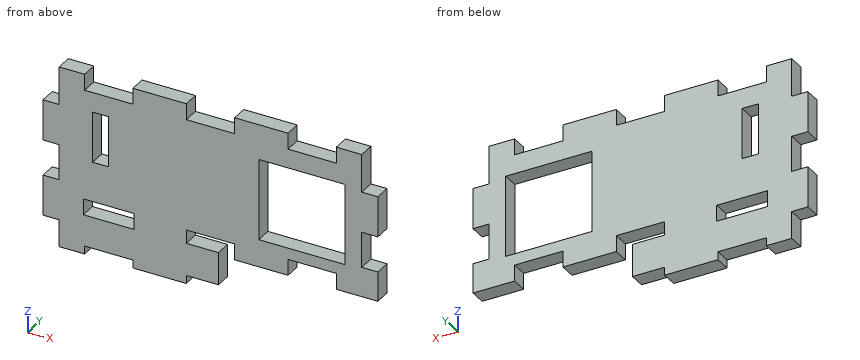
from build123d import *

# Parameters (mm, degrees)
BOTTOM_START                  = -0.928285838
BOTTOM_SIDE_PIECE_OUTLINE_W   = 3.175
BOTTOM_SIDE_PIECE_OUTLINE_H   = 10
BOTTOM_SIDE_PIECE_OUTLINE_W_2 = 10
BOTTOM_SIDE_PIECE_OUTLINE_H_2 = 3.175
BOTTOM_SIDE_PIECE_DEPTH       = 3.175
SKETCH6_W                     = 17
SKETCH6_H                     = 16
CUT_EXTRUDE2_DEPTH            = 77.155702908


# Read off the part's stored shape, not the designer's step: Bottom Side Piece
with BuildPart() as part:
    # Bottom Side Piece outline → Bottom Side Piece (new body)
    with BuildSketch(Plane(origin=(0, 0, 0), x_dir=(1, 0, 0), z_dir=(0, 1, 0)).offset(BOTTOM_START)):
        Polygon((2.240974339, 5.585190103), (5.415974339, 5.585190103), (5.415974339, -1.914809897), (10.423974339, -1.914809897), (10.423974339, 1.260190103), (19.915974339, 1.260190103), (19.915974339, -1.914809897), (30.423974339, -1.914809897), (30.423974339, 1.260190103), (39.915974339, 1.260190103), (39.915974339, -1.914809897), (50.423974339, -1.914809897), (50.423974339, 1.260190103), (59.915974339, 1.260190103), (59.915974339, -1.914809897), (64.923974339, -1.914809897), (64.923974339, 5.585190103), (68.098974339, 5.585190103), (68.098974339, 13.593190103), (64.923974339, 13.593190103), (64.923974339, 20.585190103), (68.098974339, 20.585190103), (68.098974339, 26.443190103), (59.915974339, 26.443190103), (59.915974339, 23.268190103), (50.423974339, 23.268190103), (50.423974339, 26.443190103), (39.915974339, 26.443190103), (39.915974339, 23.268190103), (30.423974339, 23.268190103), (30.423974339, 25.935190103), (36.748974339, 25.935190103), (36.748974339, 32.355690103), (30.423974339, 32.355690103), (30.423974339, 33.943190103), (19.915974339, 33.943190103), (19.915974339, 32.355690103), (10.423974339, 32.355690103), (10.423974339, 33.943190103), (5.415974339, 33.943190103), (5.415974339, 28.593190103), (2.240974339, 28.593190103), (2.240974339, 20.585190103), (5.415974339, 20.585190103), (5.415974339, 13.593190103), (2.240974339, 13.593190103), align=None)
        with Locations((13.582474339, 10.164190103)):
            Rectangle(BOTTOM_SIDE_PIECE_OUTLINE_W, BOTTOM_SIDE_PIECE_OUTLINE_H, mode=Mode.SUBTRACT)
        with Locations((56.757474339, 10.164190103)):
            Rectangle(BOTTOM_SIDE_PIECE_OUTLINE_W, BOTTOM_SIDE_PIECE_OUTLINE_H, mode=Mode.SUBTRACT)
        with Locations((15.169974339, 24.601690103)):
            Rectangle(BOTTOM_SIDE_PIECE_OUTLINE_W_2, BOTTOM_SIDE_PIECE_OUTLINE_H_2, mode=Mode.SUBTRACT)
    extrude(amount=BOTTOM_SIDE_PIECE_DEPTH)

    # Sketch6 → Cut-Extrude2 (cut, through all)
    with BuildSketch(Plane(origin=(0, 2.246714162, 0), x_dir=(1, 0, 0), z_dir=(0, 1, 0))):
        with Locations((53.169974339, 13.014190103)):
            Rectangle(SKETCH6_W, SKETCH6_H)
    extrude(amount=-CUT_EXTRUDE2_DEPTH, mode=Mode.SUBTRACT)


solid = part.part
Source: CAD feature listing. Evaluate the final solid. Frame: model axes, mm. Round coordinates to 2 decimals unless told otherwise and drop trailing zeros. Order: outer loops, then holes, each group sorted by start corner. A loop starts at its lowest first (then second) coordinate and runs counter-clockwise, first axis right, second up. Notation, with made-up numbers: (6.25, -39) -> (48.25, -39) arc R15 ccw to (48.25, -27) -> close; hole circle Ø5 at (3.5, 44). An arc over 180 degrees is marked (long way). Answer as CSV lines item,"result".
Item 1: Pin query (flat end, axial travel): pin 1 Ø1.5 at (y, z) = (1.5, -15.5) entering from +X; pin 2 Ø1.6 at (x, y) = (33.5, 0) entering from -Z; pin 3 Ø1.6 at (x, y) = (46, 0) entering from -Z. Return the tip coordinate at first contact, or that it passes through.
A:
pin 1,"x = 64.92"
pin 2,"z = -32.36"
pin 3,"z = -26.44"
Item 2: Section D-D, the plane x = 14.5. Return loops of the section in (y, z).
A:
outline,"(-0.93, -32.36) -> (2.25, -32.36) -> (2.25, -26.19) -> (-0.93, -26.19) -> close; (-0.93, -23.01) -> (2.25, -23.01) -> (2.25, -15.16) -> (-0.93, -15.16) -> close; (-0.93, -5.16) -> (2.25, -5.16) -> (2.25, -1.26) -> (-0.93, -1.26) -> close"
Item 3: Section B-B, the plane z = -17.5. Return loops of the section in (x, y).
A:
outline,"(5.42, -0.93) -> (44.67, -0.93) -> (44.67, 2.25) -> (5.42, 2.25) -> close; (61.67, -0.93) -> (64.92, -0.93) -> (64.92, 2.25) -> (61.67, 2.25) -> close"
Item 4: Line query: L1, parallel to X at y = 0.5, z = -12.5; L2, parallel to Z at x = 52.5, y = 0.35; L3, parallel to X at y = 1.85, z = -5.5. Output: solid intervals per line, ascending.
A:
L1,"2.24 to 11.99, 15.17 to 44.67, 61.67 to 68.1"
L2,"-23.27 to -21.01, -5.01 to -1.26"
L3,"5.42 to 11.99, 15.17 to 44.67, 61.67 to 64.92"
Item 5: Section A-A, the plane x = 51.5. Return loops of the section in (y, z), plus the area to 3 significant figures.
A:
outline,"(-0.93, -23.27) -> (2.25, -23.27) -> (2.25, -21.01) -> (-0.93, -21.01) -> close; (-0.93, -5.01) -> (2.25, -5.01) -> (2.25, -1.26) -> (-0.93, -1.26) -> close"
area,"19.1 mm²"
Item 6: Section C-C, the plane z = -12.5. Return loops of the section in (x, y).
A:
outline,"(2.24, -0.93) -> (11.99, -0.93) -> (11.99, 2.25) -> (2.24, 2.25) -> close; (15.17, -0.93) -> (44.67, -0.93) -> (44.67, 2.25) -> (15.17, 2.25) -> close; (61.67, -0.93) -> (68.1, -0.93) -> (68.1, 2.25) -> (61.67, 2.25) -> close"
